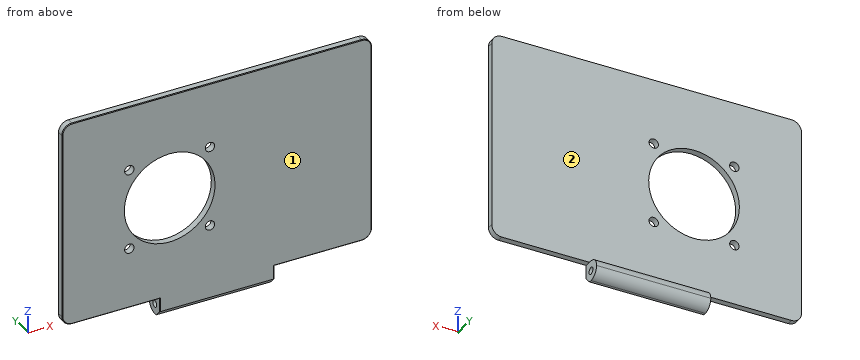
```python
from build123d import *

# Parameters (mm, degrees)
EXTRUDE_1_DEPTH     = 2
SKETCH_2_W          = 34
SKETCH_2_H          = 6
EXTRUDE_2_DEPTH     = 5.8
SKETCH_3_R          = 1.05
CUT_EXTRUDE_1_DEPTH = 93.509513024
FILLET_1_R          = 3
CHAMFER_1_SIZE      = 2
SKETCH_4_R          = 1.4
SKETCH_4_R_2        = 13.5
CUT_EXTRUDE_2_DEPTH = 2
CHAMFER_2_SIZE      = 0.2


with BuildPart() as part:
    # 草图1 → 凸台-拉伸1 (new body)
    with BuildSketch(Plane(origin=(0, 0, 0), x_dir=(1, 0, 0), z_dir=(0, 1, 0))):
        with BuildLine():
            Line((3, 0), (89.2, 0))
            ThreePointArc((89.2, 0), (91.321320344, 0.878679656), (92.2, 3))
            Line((92.2, 3), (92.2, 58.4))
            ThreePointArc((92.2, 58.4), (91.321320344, 60.521320344), (89.2, 61.4))
            Line((89.2, 61.4), (3, 61.4))
            ThreePointArc((3, 61.4), (0.878679656, 60.521320344), (0, 58.4))
            Line((0, 58.4), (0, 3))
            ThreePointArc((0, 3), (0.878679656, 0.878679656), (3, 0))
        make_face()
    extrude(amount=EXTRUDE_1_DEPTH)

    # 草图2 → 凸台-拉伸2 (add)
    with BuildSketch(Plane(origin=(0, 0, 0), x_dir=(-1, 0, 0), z_dir=(0, -1, 0))):
        with Locations((-46.1, 64.4)):
            Rectangle(SKETCH_2_W, SKETCH_2_H)
    extrude(amount=-EXTRUDE_2_DEPTH)

    # 草图3 → 切除-拉伸1 (cut, through all)
    with BuildSketch(Plane(origin=(63.1, 0, 0), x_dir=(0, 0, -1), z_dir=(1, 0, 0))):
        with Locations((64.4, 2.8)):
            Circle(SKETCH_3_R)
    extrude(amount=-CUT_EXTRUDE_1_DEPTH, mode=Mode.SUBTRACT)

    # 圆角1
    fillet_1_edges = [part.edges().sort_by_distance(p)[0] for p in [
        (46.1, 5.8, -67.4),
        (46.1, 5.8, -61.4),
    ]]
    fillet(fillet_1_edges, radius=FILLET_1_R - 0.0001)  # a hair under: the kernel refuses the full size

    # 倒角1
    chamfer_1_edges = [part.edges().sort_by_distance(p)[0] for p in [
        (46.1, 0, -67.4),
    ]]
    chamfer(chamfer_1_edges, length=CHAMFER_1_SIZE)

    # 草图4 → 切除-拉伸2 (cut)
    with BuildSketch(Plane(origin=(0, 2, 0), x_dir=(1, 0, 0), z_dir=(0, 1, 0))):
        with Locations(Location((20, 43.4, 0), (0, 0, 270))):
            Circle(SKETCH_4_R)
        with Locations(Location((44, 43.4, 0), (0, 0, 270))):
            Circle(SKETCH_4_R)
        with Locations(Location((44, 19.4, 0), (0, 0, 270))):
            Circle(SKETCH_4_R)
        with Locations(Location((20, 19.4, 0), (0, 0, 270))):
            Circle(SKETCH_4_R)
        with Locations(Location((32, 31.4, 0), (0, 0, 270))):
            Circle(SKETCH_4_R_2)
    extrude(amount=-CUT_EXTRUDE_2_DEPTH, mode=Mode.SUBTRACT)

    # 倒角2
    chamfer_2_edges = [part.edges().sort_by_distance(p)[0] for p in [
        (0, 0, -30.7),
        (0.878679656, 0, -60.521320344),
        (76.15, 0, -61.4),
        (91.321320344, 0, -60.521320344),
        (16.05, 0, -61.4),
        (29.1, 0, -63.4),
        (63.1, 0, -63.4),
        (92.2, 0, -30.7),
        (91.321320344, 0, -0.878679656),
        (46.1, 0, 0),
        (0.878679656, 0, -0.878679656),
    ]]
    chamfer(chamfer_2_edges, length=CHAMFER_2_SIZE)


solid = part.part
```
Read the model definition and answer for the solid it produces. Units are mm, in the model's axes. Face numbers are marked on the shaded views. A direction names the side the tool comes from. Coordinates: 2 decimals unless noted, no trailing zeros. Order: outer loops, then holes, each group sorted by start corner. A loop starts at its lowest first (then second) coordinate and runs counter-clockwise, first axis right, second up. Notation, with made-up numbers: (-12, -32) - (13, -32) arc R18 ccw to (13, -5) - close; hole circle Ø4 at (-24, -36.5). An arc over 180 degrees is marked (long way). Answer as a JSON object with one key per item and string values. Group by question number.
Item 1: Flat-ended cylindrical pins translate along their axes: P1, Ø2, axis at x = 11.5, y = 1.5, coming from the -Z side; P2, Ø2, axis at x = 57, z = -46, coming from the +Y side; P3, Ø0.9, axis at x = 40, y = 2.5, coming from the +Z side; P4, Ø2, axis at x = 20, z = -19.4, coming from the -Y side. Find the tip coordinate at first contact, or state that the pin passes through.
Item 2: Section B-B (z = -19.4) is taken. Give the vertices of the cut face in (x, y), plus the area to 3 significant figures.
Item 3: Section D-D (z = -27) is taken. Give the vertices of the cut face in (x, y), plus the area to 3 significant figures.
Item 4: Consider probe 1 along Y at (x, z) = (40.5, -64.4); probe 2 along X at (y, z) = (1, -19.4); probe 3 along Y at (x, z) = (46.5, -55.5). Determine where each line is inside the solid, lowest interval first. Write a range as from..to.
Item 5: Section A-A (x = 32) is taken. State how many separate pieces and enclosed holes the cut face has, plus the area to 3 significant figures.
Item 6: A tool of negligible diameter and unlimited length cuts with its end or side. For the marked faces 1 and 2, from which of +Z, -Z, +X, -X, +Y, -Y can it reach the whole face along a straight path? Write none if from no direction.
Results are:
{
 "1": {"P1": "stops at z = -61.4", "P2": "stops at y = 2", "P3": "stops at z = -61.4", "P4": "passes through"},
 "2": {"outline": "(0, 0.2) - (0.2, 0) - (18.6, 0) - (18.6, 2) - (0, 2) - close; (21.4, 0) - (25.82, 0) - (25.82, 2) - (21.4, 2) - close; (38.18, 0) - (42.6, 0) - (42.6, 2) - (38.18, 2) - close; (45.4, 0) - (92, 0) - (92.2, 0.2) - (92.2, 2) - (45.4, 2) - close", "area": "148 mm^2"},
 "3": {"outline": "(0, 0.2) - (0.2, 0) - (19.24, 0) - (19.24, 2) - (0, 2) - close; (44.76, 0) - (92, 0) - (92.2, 0.2) - (92.2, 2) - (44.76, 2) - close", "area": "133 mm^2"},
 "4": {"probe 1": "y = 0..1.75, 3.85..5.8", "probe 2": "x = 0..18.6, 21.4..25.82, 38.18..42.6, 45.4..92.2", "probe 3": "y = 0..2"},
 "5": {"separate pieces": "2", "enclosed holes": "1", "area": "94.3 mm^2"},
 "6": {"face 1": "+Z, -Z, +X, -X, -Y", "face 2": "+Z, +X, -X, +Y"}
}
